Can you work these out from the model? Positions are in its coordinate system, mm. Face numbers are marked on the shaded views. A direction names the side the tool comes from. Coordinates: 2 decimals unless noted, no trailing zeros. Loops run counter-clockwise (first coordinate to the right, second up) from the corner with the lowest first, then second, coordinate; pieces in that order, holes last. Notation, with made-up numbers: (-40, -25.75) -> (6, -25.75) arc R28 cw to (6, 12.25) -> close; hole circle Ø8 at (25.5, 47). An arc over 180 degrees is marked (long way). Put each result on its own line as item: value. Start each with the question number.
Item 1: If we section it at D-D on y = 12: Please give me the cut outline in (x, z), plus the area to 3 significant figures.
Item 2: We'd pull the mould along Z, two halves only. Please class the marked faces 4, 5 and 6: pulls with the +Z half, pulls with the -Z half, needs draft (parallel to the pull), parting line crosses it, or undercut.
Item 3: If we section it at A-A on x = 0: Please give me the cut outline in (y, z).
Item 4: Will these pins go through, and if not, where does the flat tip stop? P1, Ø4.5, axis at x = 0, z = 5, coming from the +Y side; P2, Ø10, axis at y = 10.5, z = 14, coming from the -X side; P3, Ø8, axis at y = 0, z = 15.5, coming from the -X side; P4, Ø10, axis at x = -29.5, z = 5, coming from the -Y side.
Item 5: For the marked faces 1, 2 and 3, which set-ups out of +Z, -Z, +X, -X, +Y, -Y let a thin tool reach every point of the face, with its end or its side?
Item 6: If we section it at B-B on x = -8.5: Please give me the cut outline in (y, z), plus the area to 3 significant figures.
Item 7: Please list where these lines run through material, in increasing order: L1, parallel to Z at x = 0, y = -12.1; L2, parallel to X at y = -12.7, z = 15; L3, parallel to X at y = -6, z = 10.25. Write a range as from..to.
Item 8: If we section it at C-C on z = 14.75: Please give me the cut outline in (x, y), plus the area to 3 significant figures.
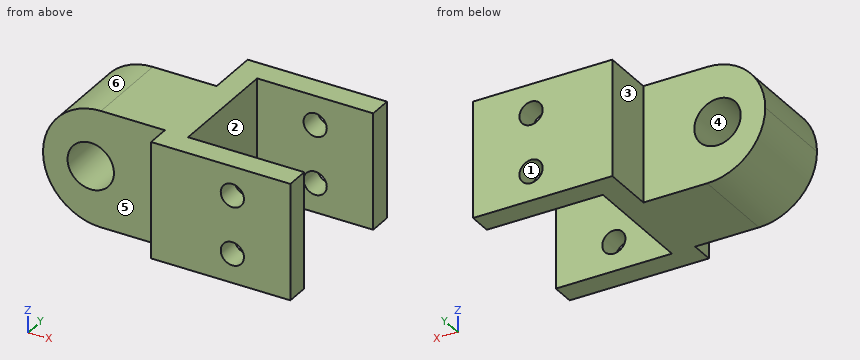
```python
from build123d import *

# Parameters (mm, degrees)
SKETCH1_W               = 25
SKETCH1_H               = 15
SKETCH1_W_2             = 20
SKETCH1_H_2             = 4
BOSS_EXTRUDE1_DEPTH     = 20
SKETCH2_R               = 4
CUT_EXTRUDE2_DEPTH      = 45.56455991
CUT_EXTRUDE3_DEPTH      = 45.56455991
CUT_EXTRUDE3_DEPTH_BACK = 45.56455991
SKETCH3_R               = 2
FILLET4_R               = 10


with BuildPart() as part:
    # Sketch1 → Boss-Extrude1 (new body)
    with BuildSketch(Plane.XY):
        with Locations((-22.5, -2.5)):
            Rectangle(SKETCH1_W, SKETCH1_H)
        Polygon((-14, 14), (-14, 5), (-10, 5), (-10, 10), (-10, 14), align=None)
        with Locations((0, 12)):
            Rectangle(SKETCH1_W_2, SKETCH1_H_2)
        Polygon((-10, -10), (-14, -10), (-14, -14), (10, -14), (10, -10), align=None)
    extrude(amount=BOSS_EXTRUDE1_DEPTH)

    # Sketch2 → Cut-Extrude2 (cut, through all)
    with BuildSketch(Plane(origin=(0, 5, 0), x_dir=(1, 0, 0), z_dir=(0, 1, 0))):
        with Locations(Location((-26.775, -10, 0), (0, 0, 270))):
            Circle(SKETCH2_R)
    extrude(amount=-CUT_EXTRUDE2_DEPTH, mode=Mode.SUBTRACT)

    # Sketch3 → Cut-Extrude3 (cut, two sides: drawn at the far end of the back side and taken through both)
    with BuildSketch(Plane(origin=(0, 5, 0), x_dir=(1, 0, 0), z_dir=(0, 1, 0)).offset(-CUT_EXTRUDE3_DEPTH_BACK)):
        with Locations(Location((0, -5, 0), (0, 0, 270))):
            Circle(SKETCH3_R)
        with Locations(Location((0, -15, 0), (0, 0, 270))):
            Circle(SKETCH3_R)
    extrude(amount=CUT_EXTRUDE3_DEPTH + CUT_EXTRUDE3_DEPTH_BACK, mode=Mode.SUBTRACT)

    # Fillet4
    fillet4_edges = [part.edges().sort_by_distance(p)[0] for p in [
        (-35, -2.5, 0),
        (-35, -2.5, 20),
    ]]
    fillet(fillet4_edges, radius=FILLET4_R - 0.0001)  # a hair under: the kernel refuses the full size


solid = part.part
```
Solutions:
1. outline: (-14, 0) -> (10, 0) -> (10, 20) -> (-14, 20) -> close; hole circle Ø4 at (0, 5); hole circle Ø4 at (0, 15)
1. area: 455 mm^2
2. face 4: undercut
2. face 5: needs draft
2. face 6: pulls with the +Z half
3. outline: (-14, 0) -> (-10, 0) -> (-10, 3) -> (-14, 3) -> close; (-14, 7) -> (-10, 7) -> (-10, 13) -> (-14, 13) -> close; (-14, 17) -> (-10, 17) -> (-10, 20) -> (-14, 20) -> close; (10, 0) -> (14, 0) -> (14, 3) -> (10, 3) -> close; (10, 7) -> (14, 7) -> (14, 13) -> (10, 13) -> close; (10, 17) -> (14, 17) -> (14, 20) -> (10, 20) -> close
4. P1: y = 14
4. P2: x = -14
4. P3: x = -34.89
4. P4: y = -10
5. face 1: +Y, -Y
5. face 2: +Z, -Z, +X
5. face 3: +Z, -Z, -X, +Y
6. outline: (-14, 0) -> (-10, 0) -> (-10, 20) -> (-14, 20) -> close; (10, 0) -> (14, 0) -> (14, 20) -> (10, 20) -> close
6. area: 160 mm^2
7. L1: 0..3, 7..13, 17..20
7. L2: -14..-2, 2..10
7. L3: -35..-30.77, -22.78..-10
8. outline: (-33.8, -10) -> (-14, -10) -> (-14, -14) -> (-1.98, -14) -> (-1.98, -10) -> (-10, -10) -> (-10, 10) -> (-1.98, 10) -> (-1.98, 14) -> (-14, 14) -> (-14, 5) -> (-33.8, 5) -> close; (1.98, -14) -> (10, -14) -> (10, -10) -> (1.98, -10) -> close; (1.98, 10) -> (10, 10) -> (10, 14) -> (1.98, 14) -> close
8. area: 537 mm^2
